from build123d import *

# Parameters (mm, degrees)
F0_R      = 25.4
F0_R_2    = 3
F1_DEPTH  = 5
F2_R      = 12
F2_R_2    = 11.1
F3_DEPTH  = 8
F4_R      = 3
F5_DEPTH  = 8.001
F9_DEPTH  = 4
F8_R      = 7
F10_DEPTH = 8.001


with BuildPart() as f1:
    # F0 (on Top) → F1 (new body)
    with BuildSketch(Plane.XY):
        Circle(F0_R)
        with BuildLine():
            ThreePointArc((-10.8845303834, -17.1589451405), (-11.8011180453, -15.6897422321), (-11.2274319001, -14.0558590249))
            Line((-11.2274319001, -14.0558590249), (-6.0965287445, -8.9249558692))
            ThreePointArc((-6.0965287445, -8.9249558692), (-5.0405306234, -8.3715104933), (-3.857237617, -8.5172893555))
            ThreePointArc((-3.857237617, -8.5172893555), (-3.5780900926, -8.638273629), (-3.295154185, -8.7501119363))
            ThreePointArc((-3.295154185, -8.7501119363), (-2.355358454, -9.4837452232), (-2, -10.6217936338))
            Line((-2, -10.6217936338), (-2, -17.8779864638))
            ThreePointArc((-2, -17.8779864638), (-2.749672532, -19.4389737228), (-4.4366812227, -19.8297317109))
            ThreePointArc((-4.4366812227, -19.8297317109), (-7.7761273457, -18.7732321006), (-10.8845303834, -17.1589451405))
        make_face(mode=Mode.SUBTRACT)
        with BuildLine():
            ThreePointArc((-19.8297317109, -4.4366812227), (-19.4389737228, -2.749672532), (-17.8779864638, -2))
            Line((-17.8779864638, -2), (-10.6217936338, -2))
            ThreePointArc((-10.6217936338, -2), (-9.4837452232, -2.355358454), (-8.7501119363, -3.295154185))
            ThreePointArc((-8.7501119363, -3.295154185), (-8.638273629, -3.5780900926), (-8.5172893555, -3.857237617))
            ThreePointArc((-8.5172893555, -3.857237617), (-8.3715104933, -5.0405306234), (-8.9249558692, -6.0965287445))
            Line((-8.9249558692, -6.0965287445), (-14.0558590249, -11.2274319001))
            ThreePointArc((-14.0558590249, -11.2274319001), (-15.6897422321, -11.8011180453), (-17.1589451405, -10.8845303834))
            ThreePointArc((-17.1589451405, -10.8845303834), (-18.7732321006, -7.7761273457), (-19.8297317109, -4.4366812227))
        make_face(mode=Mode.SUBTRACT)
        Circle(F0_R_2, mode=Mode.SUBTRACT)
        with BuildLine():
            ThreePointArc((4.4366812227, -19.8297317109), (2.749672532, -19.4389737228), (2, -17.8779864638))
            Line((2, -17.8779864638), (2, -10.6217936338))
            ThreePointArc((2, -10.6217936338), (2.355358454, -9.4837452232), (3.295154185, -8.7501119363))
            ThreePointArc((3.295154185, -8.7501119363), (3.5780900926, -8.638273629), (3.857237617, -8.5172893555))
            ThreePointArc((3.857237617, -8.5172893555), (5.0405306234, -8.3715104933), (6.0965287445, -8.9249558692))
            Line((6.0965287445, -8.9249558692), (11.2274319001, -14.0558590249))
            ThreePointArc((11.2274319001, -14.0558590249), (11.8011180453, -15.6897422321), (10.8845303834, -17.1589451405))
            ThreePointArc((10.8845303834, -17.1589451405), (7.7761273457, -18.7732321006), (4.4366812227, -19.8297317109))
        make_face(mode=Mode.SUBTRACT)
        with BuildLine():
            ThreePointArc((17.1589451405, -10.8845303834), (15.6897422321, -11.8011180453), (14.0558590249, -11.2274319001))
            Line((14.0558590249, -11.2274319001), (8.9249558692, -6.0965287445))
            ThreePointArc((8.9249558692, -6.0965287445), (8.3715104933, -5.0405306234), (8.5172893555, -3.857237617))
            ThreePointArc((8.5172893555, -3.857237617), (8.638273629, -3.5780900926), (8.7501119363, -3.295154185))
            ThreePointArc((8.7501119363, -3.295154185), (9.4837452232, -2.355358454), (10.6217936338, -2))
            Line((10.6217936338, -2), (17.8779864638, -2))
            ThreePointArc((17.8779864638, -2), (19.4389737228, -2.749672532), (19.8297317109, -4.4366812227))
            ThreePointArc((19.8297317109, -4.4366812227), (18.7732321006, -7.7761273457), (17.1589451405, -10.8845303834))
        make_face(mode=Mode.SUBTRACT)
        with BuildLine():
            ThreePointArc((-17.1589451405, 10.8845303834), (-15.6897422321, 11.8011180453), (-14.0558590249, 11.2274319001))
            Line((-14.0558590249, 11.2274319001), (-8.9249558692, 6.0965287445))
            ThreePointArc((-8.9249558692, 6.0965287445), (-8.3715104933, 5.0405306234), (-8.5172893555, 3.857237617))
            ThreePointArc((-8.5172893555, 3.857237617), (-8.638273629, 3.5780900926), (-8.7501119363, 3.295154185))
            ThreePointArc((-8.7501119363, 3.295154185), (-9.4837452232, 2.355358454), (-10.6217936338, 2))
            Line((-10.6217936338, 2), (-17.8779864638, 2))
            ThreePointArc((-17.8779864638, 2), (-19.4389737228, 2.749672532), (-19.8297317109, 4.4366812227))
            ThreePointArc((-19.8297317109, 4.4366812227), (-18.7732321006, 7.7761273457), (-17.1589451405, 10.8845303834))
        make_face(mode=Mode.SUBTRACT)
        with BuildLine():
            ThreePointArc((-10.8845303834, 17.1589451405), (-7.7761273457, 18.7732321006), (-4.4366812227, 19.8297317109))
            ThreePointArc((-4.4366812227, 19.8297317109), (-2.749672532, 19.4389737228), (-2, 17.8779864638))
            Line((-2, 17.8779864638), (-2, 10.6217936338))
            ThreePointArc((-2, 10.6217936338), (-2.355358454, 9.4837452232), (-3.295154185, 8.7501119363))
            ThreePointArc((-3.295154185, 8.7501119363), (-3.5780900926, 8.638273629), (-3.857237617, 8.5172893555))
            ThreePointArc((-3.857237617, 8.5172893555), (-5.0405306234, 8.3715104933), (-6.0965287445, 8.9249558692))
            Line((-6.0965287445, 8.9249558692), (-11.2274319001, 14.0558590249))
            ThreePointArc((-11.2274319001, 14.0558590249), (-11.8011180453, 15.6897422321), (-10.8845303834, 17.1589451405))
        make_face(mode=Mode.SUBTRACT)
        with BuildLine():
            ThreePointArc((19.8297317109, 4.4366812227), (19.4389737228, 2.749672532), (17.8779864638, 2))
            Line((17.8779864638, 2), (10.6217936338, 2))
            ThreePointArc((10.6217936338, 2), (9.4837452232, 2.355358454), (8.7501119363, 3.295154185))
            ThreePointArc((8.7501119363, 3.295154185), (8.638273629, 3.5780900926), (8.5172893555, 3.857237617))
            ThreePointArc((8.5172893555, 3.857237617), (8.3715104933, 5.0405306234), (8.9249558692, 6.0965287445))
            Line((8.9249558692, 6.0965287445), (14.0558590249, 11.2274319001))
            ThreePointArc((14.0558590249, 11.2274319001), (15.6897422321, 11.8011180453), (17.1589451405, 10.8845303834))
            ThreePointArc((17.1589451405, 10.8845303834), (18.7732321006, 7.7761273457), (19.8297317109, 4.4366812227))
        make_face(mode=Mode.SUBTRACT)
        with BuildLine():
            Line((2, 10.6217936338), (2, 17.8779864638))
            ThreePointArc((2, 17.8779864638), (2.749672532, 19.4389737228), (4.4366812227, 19.8297317109))
            ThreePointArc((4.4366812227, 19.8297317109), (7.7761273457, 18.7732321006), (10.8845303834, 17.1589451405))
            ThreePointArc((10.8845303834, 17.1589451405), (11.8011180453, 15.6897422321), (11.2274319001, 14.0558590249))
            Line((11.2274319001, 14.0558590249), (6.0965287445, 8.9249558692))
            ThreePointArc((6.0965287445, 8.9249558692), (5.0405306234, 8.3715104933), (3.857237617, 8.5172893555))
            ThreePointArc((3.857237617, 8.5172893555), (3.5780900926, 8.638273629), (3.295154185, 8.7501119363))
            ThreePointArc((3.295154185, 8.7501119363), (2.355358454, 9.4837452232), (2, 10.6217936338))
        make_face(mode=Mode.SUBTRACT)
    extrude(amount=F1_DEPTH)

    # F2 (on Top) → F3 (join)
    with BuildSketch(Plane.XY):
        Circle(F2_R)
        Circle(F2_R_2, mode=Mode.SUBTRACT)
    extrude(amount=F3_DEPTH)

    # F4 (on face) → F5 (cut, through all)
    with BuildSketch(Plane.XY.offset(8)):
        Circle(F4_R)
    extrude(amount=-F5_DEPTH, mode=Mode.SUBTRACT)

    # F6 (on Right) → F7 (revolve, cut)
    with BuildSketch(Plane.YZ):
        Polygon((25.4579713509, 0.9026185274), (25.4, 2.4026185274), (23.4, 2.4026185274), align=None)
        Polygon((23.4, 2.4026185274), (25.4, 2.4026185274), (25.4579713509, 3.9026185274), align=None)
    revolve(axis=Axis((0, 0, 8.0988456029), (0, 0, -1)), mode=Mode.SUBTRACT)

    # F9 (cut): a face of the model
    f9_faces = [f1.faces().sort_by_distance(p)[0] for p in [
        (-7.6268852712, -7.6268852712, 5),
    ]]
    extrude(f9_faces, amount=-F9_DEPTH, mode=Mode.SUBTRACT)

    # F8 (on Top) → F10 (cut, through all)
    with BuildSketch(Plane.XY):
        Circle(F8_R)
    extrude(amount=F10_DEPTH, mode=Mode.SUBTRACT)


solid = f1.part
Geometry check sheet. Reference: the model listing, model coordinates, mm. A direction names the side the tool comes from. Give positions to 0.01 mm unless a question says otherwise; leave off trailing zeros.
1) Cross-section at A-A (x = 13). Count the separate pieces of the cut face and the enclosed holes in it, plus the area to 3 significant figures.
Values follow:
separate pieces: 3
enclosed holes: 0
area: 130 mm2
2) Release check for a two-part mould opening along X. For faces 1 (the face through (6.466, -2.681, 0.493)), 2 (the face through (-18.792, 7.731, 2.465)), 3 (the face through (-5.506, -24.796, 0.466)), 4 (the face through (5.3, -5.3, 0)) record: released by +X, released by -X, zero draft, split by the parting line, or undercut.
Values follow:
face 1: undercut
face 2: undercut
face 3: split by the parting line
face 4: zero draft
3) Set-up check for faces 5 (the face through (-9.47, 2.365, 0.493)), 6 (the face through (11, -11, 5)): record each of +Z, -Z, +X, -X, +Y, -Y from which the full face is reachable in a straight line by a thin tool's end or side.
Values follow:
face 5: +Z, -Z
face 6: +Z
4) Thickness scan on line 1 (Y direction, x = 0, z = 5.25); line 2 (X direction, y = 0, z = 0.5); line 3 (X direction, y = -11, z = 0.75). Record the ranges inside material, lowest first.
Values follow:
line 1: y = -12 to -11.1, 11.1 to 12
line 2: x = -25.4 to -7, 7 to 25.4
line 3: x = -22.89 to -17.08, -13.83 to -8.17, -4.8 to 4.8, 8.17 to 13.83, 17.08 to 22.89
5) Go/stop test with flat-tipped pins: pin 1 Ø2.5 at (x, z) = (15.5, 3.5) entering from +Y; pin 2 Ø1.5 at (y, z) = (-16.5, 6) entering from -X; pin 3 Ø10 at (x, y) = (-5, -8.5) entering from -Z; pin 4 Ø1.5 at (y, z) = (-14.5, 3) entering from -X. Record where each tip stops, or that it passes through.
Values follow:
pin 1: stops at y = 20.99
pin 2: passes through
pin 3: stops at z = 0
pin 4: stops at x = -20.77
